Answer from the drawing. Dimensions are ordinates in mm from the lowest x, y and z of the part. Coordinates: 2 decimals unless noted, no trailing zeros. Order: outer loops, then holes, each group sorted by start corner. A loop starts at its lowest first (then second) coordinate and runs counter-clockwise, first axis right, second up. Notation, with made-up numbers: (6.25, -23) - (59.25, -23) arc R35 ccw to (59.25, 15) - close; hole circle Ø8 at (70.5, 20.25). An arc over 180 degrees is marked (long way). Use a Markdown table: item, result. Add a question column.
Item 1: Flat-ended cylindrical pins translate along their axes: P1, Ø1.5, axis at x = 568, y = 12.5, coming from the -Z side; P2, Ø3, axis at x = 308, y = 9, coming from the -Z side; P3, Ø2, axis at y = 5.5, z = 201, coming from the -X side. Find the tip coordinate at first contact, or state that the pin passes through.
Item 2: The part is cut by section B-B, the plane y = 6.25. Give the vertices of the cut face in (x, z).
Item 3: The part is cut by section A-A, the plane x = 659.5. Give the vertices of the cut face in (y, z), then the cut area to 3 significant figures.
Item 4: Find the intervals of material crossed by line 1 along Z through (x, y) = (168.5, 11.25); line 2 along X through (y, z) = (3.25, 75.5), in increasing order.
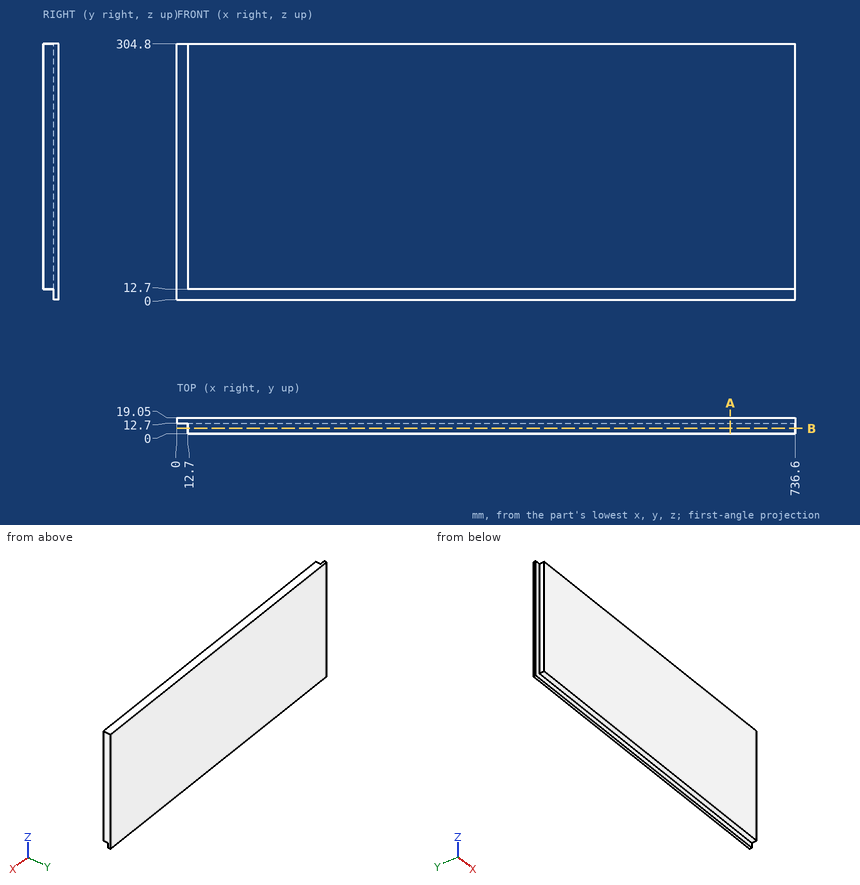
Solution:
| question | item | result |
|---|---|---|
| 1 | P1 | stops at z = 0 |
| 1 | P2 | stops at z = 12.7 |
| 1 | P3 | stops at x = 12.7 |
| 2 | outline | (12.7, 12.7) - (736.6, 12.7) - (736.6, 304.8) - (12.7, 304.8) - close |
| 3 | outline | (0, 12.7) - (12.7, 12.7) - (12.7, 0) - (19.05, 0) - (19.05, 304.8) - (0, 304.8) - close |
| 3 | area | 5,650 mm2 |
| 4 | line 1 | z = 12.7 to 304.8 |
| 4 | line 2 | x = 12.7 to 736.6 |
